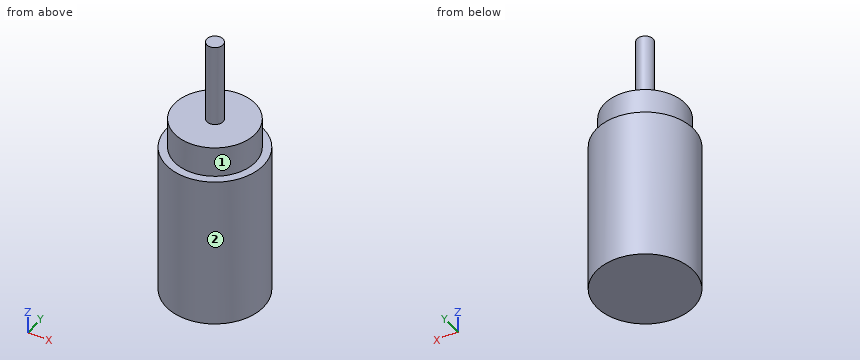
Autodesk Inventor part; units mm, degrees
ref_plane "YZ Plane" through (0, 0, 0) normal (1, 0, 0) x (0, 1, 0)
ref_plane "XZ Plane" through (0, 0, 0) normal (0, 1, 0) x (-1, 0, 0)
ref_plane "XY Plane" through (0, 0, 0) normal (0, 0, 1) x (1, 0, 0)
sketch "Sketch1" plane through (0, 0, 0) normal (0, 0, 1) x (1, 0, 0)
  circle A0 centre (0, 0) radius 3
  dimension "d0" = 6
extrude "Extrusion1" add sketch "Sketch1" along normal mid plane 9.5
sketch "Sketch2" plane through (0, 0, 4.75) normal (0, 0, 1) x (1, 0, 0)
  circle A0 centre (0, 0) radius 2.5
  dimension "d3" = 5
extrude "Extrusion2" add sketch "Sketch2" along normal blind 1.9
sketch "Sketch3" plane through (0, 0, 6.65) normal (0, 0, 1) x (1, 0, 0)
  circle A0 centre (0, 0) radius 0.5
  dimension "d6" = 1
extrude "Extrusion3" add sketch "Sketch3" along normal blind 5.15
properties part number "FDM0620 Stepper"
Can you work these out from the model? Positions are in its coordinate system, mm. Face numbers are marked on the shaded views. A direction names the side the tool comes from. Round coordinates to 2 decimals unless told otherwise and drop trailing zeros. Loops run counter-clockwise (first coordinate to the right, second up) from the corner with the lowest first, then second, coordinate; pieces in that order, holes last. Notation, with made-up numbers: M 33,56 L 83,56 A36 cw 83,93 Z; hole C -20.5,67.25 d1. An arc over 180 degrees is marked long. Answer in a Markdown table with one row per item.
1. If we section it at A-A, the plane y = 0: Please give me the cut outline in (x, z), plus the area to 4 significant figures.
Established:
| item | result |
|---|---|
| outline | M -3,-4.75 L 3,-4.75 L 3,4.75 L 2.5,4.75 L 2.5,6.65 L 0.5,6.65 L 0.5,11.8 L -0.5,11.8 L -0.5,6.65 L -2.5,6.65 L -2.5,4.75 L -3,4.75 Z |
| area | 71.65 mm² |
2. If we section it at D-D, the plane y = -1.1: Please give me the cut outline in (x, z) (3 decimals), plus the area to 3 significant figures.
Established:
| item | result |
|---|---|
| outline | M -2.791,-4.75 L 2.791,-4.75 L 2.791,4.75 L 2.245,4.75 L 2.245,6.65 L -2.245,6.65 L -2.245,4.75 L -2.791,4.75 Z |
| area | 61.6 mm² |
3. I'm going to push flat-ended pins straight in: pin 1 Ø1 at (y, z) = (2, 0.5) entering from +X; pin 2 Ø1 at (x, z) = (1, 6) entering from -Y. Where does each tip first touch, or does it pass through?
Established:
| item | result |
|---|---|
| pin 1 | x = 2.6 |
| pin 2 | y = -2.45 |
4. On a 3-axis mill with a long thin cutter (end or side, diameter ignored), from which of +Z, -Z, +X, -X, +Y, -Y can I reach the whole of each face in a straight line? I mean the marked faces 1 and 2. Say none if no direction works.
Established:
| item | result |
|---|---|
| face 1 | +Z |
| face 2 | +Z, -Z |
5. Please list where these lines run through material, in increasing order: line 1 (Z direction, x = -1.65, y = 2.45); line 2 (Z direction, x = 1.75, y = 0.25); line 3 (X direction, y = -0.1, z = 6.5). Write a range as from..to.
Established:
| item | result |
|---|---|
| line 1 | -4.75..4.75 |
| line 2 | -4.75..6.65 |
| line 3 | -2.5..2.5 |
6. If we section it at C-C, the plane z = 10: Please give me the cut outline in (x, y).
Established:
| item | result |
|---|---|
| outline | C 0,0 d1 |
